from build123d import *

# Parameters (mm, degrees)
SKETCH_1_W              = 10
SKETCH_1_H              = 2
SKETCH_2_R              = 4.5
EXTRUDE_1_DEPTH         = 2.5
CUT_EXTRUDE_1_DEPTH     = 3.6
HOLE_WIZARD_3_0_3_1_D   = 3
HOLE_WIZARD_2_5_2_5_1_D = 2.5
CHAMFER_1_SIZE          = 0.140560122
CHAMFER_1_EDGE_2_SIZE   = 0.140560122
CHAMFER_1_EDGE_3_SIZE   = 0.140560122
CHAMFER_1_EDGE_4_SIZE   = 0.140560122
CHAMFER_1_EDGE_5_SIZE   = 0.140560122
CHAMFER_1_EDGE_6_SIZE   = 0.140560122
CHAMFER_1_EDGE_7_SIZE   = 0.140560122
CHAMFER_1_EDGE_8_SIZE   = 0.140560122
CHAMFER_1_EDGE_9_SIZE   = 0.140560122
CHAMFER_1_EDGE_10_SIZE  = 0.140560122
CHAMFER_1_EDGE_11_SIZE  = 0.140560122
CHAMFER_1_EDGE_12_SIZE  = 0.140560122
CHAMFER_1_EDGE_13_SIZE  = 0.140560122
CHAMFER_1_EDGE_14_SIZE  = 0.140560122
CHAMFER_1_EDGE_15_SIZE  = 0.140560122
CHAMFER_1_EDGE_16_SIZE  = 0.140560122
CHAMFER_1_EDGE_17_SIZE  = 0.140560122
CHAMFER_1_EDGE_18_SIZE  = 0.140560122
CHAMFER_1_EDGE_19_SIZE  = 0.140560122
CHAMFER_1_EDGE_20_SIZE  = 0.140560122
CHAMFER_1_EDGE_21_SIZE  = 0.140560122
CHAMFER_1_EDGE_22_SIZE  = 0.140560122
CHAMFER_1_EDGE_23_SIZE  = 0.140560122
CHAMFER_1_EDGE_24_SIZE  = 0.140560122
CHAMFER_1_EDGE_25_SIZE  = 0.140560122
CHAMFER_1_EDGE_26_SIZE  = 0.140560122
SKETCH_8_R              = 4.5
CUT_EXTRUDE_2_DEPTH     = 4.5
SKETCH_9_R              = 4.5
SKETCH_9_R_2            = 3.15
EXTRUDE_2_DEPTH         = 2


with BuildPart() as part:
    # Эскиз1 → Повернуть1 (revolve)
    with BuildSketch(Plane.XY, mode=Mode.PRIVATE) as revolve_1_sk:
        with Locations((5, 1)):
            Rectangle(SKETCH_1_W, SKETCH_1_H)
    revolve(revolve_1_sk.sketch.rotate(Axis((0, 2, 0), (0, -1, 0)), 270), axis=Axis((0, 2, 0), (0, -1, 0)))

    # Эскиз2 → Бобышка-Вытянуть1 (add)
    with BuildSketch(Plane(origin=(0, 2, 0), x_dir=(-1, 0, 0), z_dir=(0, 1, 0))):
        with Locations(Location((0, 0, 0), (0, 0, 90))):
            Circle(SKETCH_2_R)
    extrude(amount=EXTRUDE_1_DEPTH)

    # Эскиз3 → Вырез-Вытянуть1 (cut)
    with BuildSketch(Plane(origin=(0, 4.5, 0), x_dir=(-1, 0, 0), z_dir=(0, 1, 0))):
        Polygon((-2.711547104, 1.028354172), (-2.477853855, 0.610736123), (-2.878855735, 0.349556373), (-2.552010646, 0), (-2.878855735, -0.349556373), (-2.477853855, -0.610736123), (-2.711547104, -1.028354172), (-2.259693204, -1.185978483), (-2.386653211, -1.647387766), (-1.910207398, -1.692296084), (-1.923055709, -2.17068117), (-1.449707281, -2.100263587), (-1.347697199, -2.567822474), (-0.904955447, -2.386171406), (-0.694015426, -2.815731271), (-0.307610891, -2.533403615), (0, -2.9), (0.307610891, -2.533403615), (0.694015426, -2.815731271), (0.904955447, -2.386171406), (1.347697199, -2.567822474), (1.449707281, -2.100263587), (1.923055709, -2.17068117), (1.910207398, -1.692296084), (2.386653211, -1.647387766), (2.259693204, -1.185978483), (2.711547104, -1.028354172), (2.477853855, -0.610736123), (2.878855735, -0.349556373), (2.552010646, 0), (2.878855735, 0.349556373), (2.477853855, 0.610736123), (2.711547104, 1.028354172), (2.259693204, 1.185978483), (2.386653211, 1.647387766), (1.910207398, 1.692296084), (1.923055709, 2.17068117), (1.449707281, 2.100263587), (1.347697199, 2.567822474), (0.904955447, 2.386171406), (0.694015426, 2.815731271), (0.307610891, 2.533403615), (0, 2.9), (-0.307610891, 2.533403615), (-0.694015426, 2.815731271), (-0.904955447, 2.386171406), (-1.347697199, 2.567822474), (-1.449707281, 2.100263587), (-1.923055709, 2.17068117), (-1.910207398, 1.692296084), (-2.386653211, 1.647387766), (-2.259693204, 1.185978483), align=None)
    extrude(amount=-CUT_EXTRUDE_1_DEPTH, mode=Mode.SUBTRACT)

    # Диаметр отверстия Ø3.0 (3)1 (through all)
    with Locations(Plane(origin=(0, 0.9, 0), x_dir=(1, 0, 0), z_dir=(0, 1, 0))):
        with Locations((0, 0)):
            Hole(HOLE_WIZARD_3_0_3_1_D / 2)

    # Диаметр отверстия Ø2.5 (2.5)1 (through all)
    with Locations(Plane(origin=(0, 2, 0), x_dir=(1, 0, 0), z_dir=(0, 1, 0))):
        with Locations((-4.949747468, 4.949747468), (4.949747468, 4.949747468), (4.949747468, -4.949747468), (-4.949747468, -4.949747468)):
            Hole(HOLE_WIZARD_2_5_2_5_1_D / 2)

    # Фаска1
    chamfer_1_edges = [part.edges().sort_by_distance(p)[0] for p in [
        (2.259693204, 2.7, 1.185978483),
    ]]
    chamfer(chamfer_1_edges, length=CHAMFER_1_SIZE)

    # Фаска1 edge 2
    chamfer_1_edge_2_edges = [part.edges().sort_by_distance(p)[0] for p in [
        (1.910207398, 2.7, 1.692296084),
    ]]
    chamfer(chamfer_1_edge_2_edges, length=CHAMFER_1_EDGE_2_SIZE)

    # Фаска1 edge 3
    chamfer_1_edge_3_edges = [part.edges().sort_by_distance(p)[0] for p in [
        (1.449707281, 2.7, 2.100263587),
    ]]
    chamfer(chamfer_1_edge_3_edges, length=CHAMFER_1_EDGE_3_SIZE)

    # Фаска1 edge 4
    chamfer_1_edge_4_edges = [part.edges().sort_by_distance(p)[0] for p in [
        (0.904955447, 2.7, 2.386171406),
    ]]
    chamfer(chamfer_1_edge_4_edges, length=CHAMFER_1_EDGE_4_SIZE)

    # Фаска1 edge 5
    chamfer_1_edge_5_edges = [part.edges().sort_by_distance(p)[0] for p in [
        (0.307610891, 2.7, 2.533403615),
    ]]
    chamfer(chamfer_1_edge_5_edges, length=CHAMFER_1_EDGE_5_SIZE)

    # Фаска1 edge 6
    chamfer_1_edge_6_edges = [part.edges().sort_by_distance(p)[0] for p in [
        (-0.307610891, 2.7, 2.533403615),
    ]]
    chamfer(chamfer_1_edge_6_edges, length=CHAMFER_1_EDGE_6_SIZE)

    # Фаска1 edge 7
    chamfer_1_edge_7_edges = [part.edges().sort_by_distance(p)[0] for p in [
        (-0.904955447, 2.7, 2.386171406),
    ]]
    chamfer(chamfer_1_edge_7_edges, length=CHAMFER_1_EDGE_7_SIZE)

    # Фаска1 edge 8
    chamfer_1_edge_8_edges = [part.edges().sort_by_distance(p)[0] for p in [
        (-1.449707281, 2.7, 2.100263587),
    ]]
    chamfer(chamfer_1_edge_8_edges, length=CHAMFER_1_EDGE_8_SIZE)

    # Фаска1 edge 9
    chamfer_1_edge_9_edges = [part.edges().sort_by_distance(p)[0] for p in [
        (-1.910207398, 2.7, 1.692296084),
    ]]
    chamfer(chamfer_1_edge_9_edges, length=CHAMFER_1_EDGE_9_SIZE)

    # Фаска1 edge 10
    chamfer_1_edge_10_edges = [part.edges().sort_by_distance(p)[0] for p in [
        (-2.259693204, 2.7, 1.185978483),
    ]]
    chamfer(chamfer_1_edge_10_edges, length=CHAMFER_1_EDGE_10_SIZE)

    # Фаска1 edge 11
    chamfer_1_edge_11_edges = [part.edges().sort_by_distance(p)[0] for p in [
        (-2.477853855, 2.7, 0.610736123),
    ]]
    chamfer(chamfer_1_edge_11_edges, length=CHAMFER_1_EDGE_11_SIZE)

    # Фаска1 edge 12
    chamfer_1_edge_12_edges = [part.edges().sort_by_distance(p)[0] for p in [
        (-2.552010646, 2.7, 0),
    ]]
    chamfer(chamfer_1_edge_12_edges, length=CHAMFER_1_EDGE_12_SIZE)

    # Фаска1 edge 13
    chamfer_1_edge_13_edges = [part.edges().sort_by_distance(p)[0] for p in [
        (-2.477853855, 2.7, -0.610736123),
    ]]
    chamfer(chamfer_1_edge_13_edges, length=CHAMFER_1_EDGE_13_SIZE)

    # Фаска1 edge 14
    chamfer_1_edge_14_edges = [part.edges().sort_by_distance(p)[0] for p in [
        (-2.259693204, 2.7, -1.185978483),
    ]]
    chamfer(chamfer_1_edge_14_edges, length=CHAMFER_1_EDGE_14_SIZE)

    # Фаска1 edge 15
    chamfer_1_edge_15_edges = [part.edges().sort_by_distance(p)[0] for p in [
        (-1.910207398, 2.7, -1.692296084),
    ]]
    chamfer(chamfer_1_edge_15_edges, length=CHAMFER_1_EDGE_15_SIZE)

    # Фаска1 edge 16
    chamfer_1_edge_16_edges = [part.edges().sort_by_distance(p)[0] for p in [
        (-1.449707281, 2.7, -2.100263587),
    ]]
    chamfer(chamfer_1_edge_16_edges, length=CHAMFER_1_EDGE_16_SIZE)

    # Фаска1 edge 17
    chamfer_1_edge_17_edges = [part.edges().sort_by_distance(p)[0] for p in [
        (-0.904955447, 2.7, -2.386171406),
    ]]
    chamfer(chamfer_1_edge_17_edges, length=CHAMFER_1_EDGE_17_SIZE)

    # Фаска1 edge 18
    chamfer_1_edge_18_edges = [part.edges().sort_by_distance(p)[0] for p in [
        (-0.307610891, 2.7, -2.533403615),
    ]]
    chamfer(chamfer_1_edge_18_edges, length=CHAMFER_1_EDGE_18_SIZE)

    # Фаска1 edge 19
    chamfer_1_edge_19_edges = [part.edges().sort_by_distance(p)[0] for p in [
        (0.307610891, 2.7, -2.533403615),
    ]]
    chamfer(chamfer_1_edge_19_edges, length=CHAMFER_1_EDGE_19_SIZE)

    # Фаска1 edge 20
    chamfer_1_edge_20_edges = [part.edges().sort_by_distance(p)[0] for p in [
        (0.904955447, 2.7, -2.386171406),
    ]]
    chamfer(chamfer_1_edge_20_edges, length=CHAMFER_1_EDGE_20_SIZE)

    # Фаска1 edge 21
    chamfer_1_edge_21_edges = [part.edges().sort_by_distance(p)[0] for p in [
        (1.449707281, 2.7, -2.100263587),
    ]]
    chamfer(chamfer_1_edge_21_edges, length=CHAMFER_1_EDGE_21_SIZE)

    # Фаска1 edge 22
    chamfer_1_edge_22_edges = [part.edges().sort_by_distance(p)[0] for p in [
        (1.910207398, 2.7, -1.692296084),
    ]]
    chamfer(chamfer_1_edge_22_edges, length=CHAMFER_1_EDGE_22_SIZE)

    # Фаска1 edge 23
    chamfer_1_edge_23_edges = [part.edges().sort_by_distance(p)[0] for p in [
        (2.259693204, 2.7, -1.185978483),
    ]]
    chamfer(chamfer_1_edge_23_edges, length=CHAMFER_1_EDGE_23_SIZE)

    # Фаска1 edge 24
    chamfer_1_edge_24_edges = [part.edges().sort_by_distance(p)[0] for p in [
        (2.477853855, 2.7, -0.610736123),
    ]]
    chamfer(chamfer_1_edge_24_edges, length=CHAMFER_1_EDGE_24_SIZE)

    # Фаска1 edge 25
    chamfer_1_edge_25_edges = [part.edges().sort_by_distance(p)[0] for p in [
        (2.552010646, 2.7, 0),
    ]]
    chamfer(chamfer_1_edge_25_edges, length=CHAMFER_1_EDGE_25_SIZE)

    # Фаска1 edge 26
    chamfer_1_edge_26_edges = [part.edges().sort_by_distance(p)[0] for p in [
        (2.477853855, 2.7, 0.610736123),
    ]]
    chamfer(chamfer_1_edge_26_edges, length=CHAMFER_1_EDGE_26_SIZE)

    # Эскиз8 → Вырез-Вытянуть2 (cut)
    with BuildSketch(Plane(origin=(0, 4.5, 0), x_dir=(1, 0, 0), z_dir=(0, 1, 0))):
        with Locations(Location((0, 0, 0), (0, 0, 270))):
            Circle(SKETCH_8_R)
    extrude(amount=-CUT_EXTRUDE_2_DEPTH, mode=Mode.SUBTRACT)

    # Эскиз9 → Бобышка-Вытянуть2 (add)
    with BuildSketch(Plane.XZ):
        Circle(SKETCH_9_R)
        with Locations(Location((0, 0, 0), (0, 0, 270))):
            Circle(SKETCH_9_R_2, mode=Mode.SUBTRACT)
    extrude(amount=-EXTRUDE_2_DEPTH)


solid = part.part
Input: part model. Units: mm. Frame: model coordinates. Coordinates: 2 decimals unless noted, no trailing zeros. Loops run counter-clockwise (first coordinate to the right, second up) from the corner with the lowest first, then second, coordinate; pieces in that order, holes last. Notation, with made-up numbers: (38, -12.5) - (57, -12.5) arc R15 cw to (57, -5.5) - close; hole circle Ø7 at (89.25, -36.5). An arc over 180 degrees is marked (long way). Answer in a Markdown table with one row per item. Add a question column.
Item 1: Mould query, pull axis X, two halves, no side actions, for faces 1 (the flat face through (-2.4, 2, 2.4)), 2 (the cylindrical face through (-9.76, 1.01, 2.17)), 3 (the cylindrical face through (-4.68, 0.99, -3.73)). Classes: released by +X, released by -X, zero draft, split by the parting line, or undercut.
Item 2: Contact query for a flat-ended pin moving along its axis: P1, Ø5.5, axis at x = 0, z = 0, coming from the -Y side. Output: stop coordinate, or through.
Item 3: Section query C-C on x = 5. Return the cut outline in (y, z).
Item 4: Line query: line 1 along X through (y, z) = (1, -4.25); line 2 along X through (y, z) = (1.8, 5.25). Output: solid intervals per line, ascending. Write a range as [from, to].
Item 5: Section query B-B on z = 0. Return the cut outline in (x, y), then the cut area to 3 significant figures.
Item 6: Section query A-A on x = 0. Return the cut outline in (y, z), then the cut area to 3 significant figures.
Item 7: Section query D-D on z = 5.5. Return the cut outline in (x, y).
Recorded:
| question | item | result |
|---|---|---|
| 1 | face 1 | zero draft |
| 1 | face 2 | split by the parting line |
| 1 | face 3 | undercut |
| 2 | P1 | through |
| 3 | outline | (0, -8.66) - (2, -8.66) - (2, -6.2) - (0, -6.2) - close; (0, -3.7) - (2, -3.7) - (2, 3.7) - (0, 3.7) - close; (0, 6.2) - (2, 6.2) - (2, 8.66) - (0, 8.66) - close |
| 4 | line 1 | [-9.05, -5.99], [-3.91, 3.91], [5.99, 9.05] |
| 4 | line 2 | [-8.51, -6.16], [-3.74, 3.74], [6.16, 8.51] |
| 5 | outline | (-10, 0) - (-3.15, 0) - (-3.15, 2) - (-10, 2) - close; (3.15, 0) - (10, 0) - (10, 2) - (3.15, 2) - close |
| 5 | area | 27.4 mm^2 |
| 6 | outline | (0, -10) - (2, -10) - (2, -3.15) - (0, -3.15) - close; (0, 3.15) - (2, 3.15) - (2, 10) - (0, 10) - close |
| 6 | area | 27.4 mm^2 |
| 7 | outline | (-8.35, 0) - (-6.07, 0) - (-6.07, 2) - (-8.35, 2) - close; (-3.83, 0) - (3.83, 0) - (3.83, 2) - (-3.83, 2) - close; (6.07, 0) - (8.35, 0) - (8.35, 2) - (6.07, 2) - close |
